Input: dimensioned drawing with shaded views. Units: mm. Origin: part minimum x, y, z. A direction names the side the tool comes from. Round coordinates to 2 decimals unless told otherwise and drop trailing zeros. Loops run counter-clockwise (first coordinate to the right, second up) from the corner with the lowest first, then second, coordinate; pieces in that order, holes last. Notation, with made-up numbers: M 5.5,-29.75 L 54.5,-29.75 A14 ccw 54.5,-14.75 Z; hole C -24,31.5 d3. An arc over 180 degrees is marked long. Use one line per item in the form item = value. Start each with the question number.
Q1. Section query B-B, the plane y = 33. Output: boundary loops of the cut face in (x, z), and give its area (3 significant figures).
Q2. Section query C-C, the plane z = 3.1. Output: boundary loops of the cut face in (x, y), and give its area (3 significant figures).
Q3. First-contact query: P1, Ø3, axis at x = 31.5, z = 2.5, coming from the -Y side; P2, Ø1.5, axis at y = 71.5, z = 3, coming from the -X side; P3, Ø2.5, axis at x = 38, z = 1.5, coming from the -Y side. Flat tips, straight axial feed; report the tip coordinate or a pass-through.
Q4. Ray query, line 1 along Y through (x, z) = (17.5, 3.9); line 2 along Y through (x, z) = (14, 2.7); line 3 along X through (y, z) = (36, 1.95). Return the intervals inside material, ascending.
Q5. Section query D-D, the plane y = 20. Output: boundary loops of the cut face in (x, z).
Q6. Section query A-A, the plane x = 17.5. Output: boundary loops of the cut face in (y, z), and give its area (3 significant figures).
Q7. Access query for the marked faces 1, 2, 3, 4 and 5. Directions: +Z, -Z, +X, -X, +Y, -Y. A direction counts if a zero-diameter tool reaches every point of the face in a straight line with its end or side. Return the directions, or none.
Q8. Mould query, pull axis X, two halves, no side actions, for the marked faces 6, 7 and 8. Classes: pulls with the +X half, pulls with the -X half, needs draft (parallel to the pull), parting line crosses it, or undercut.
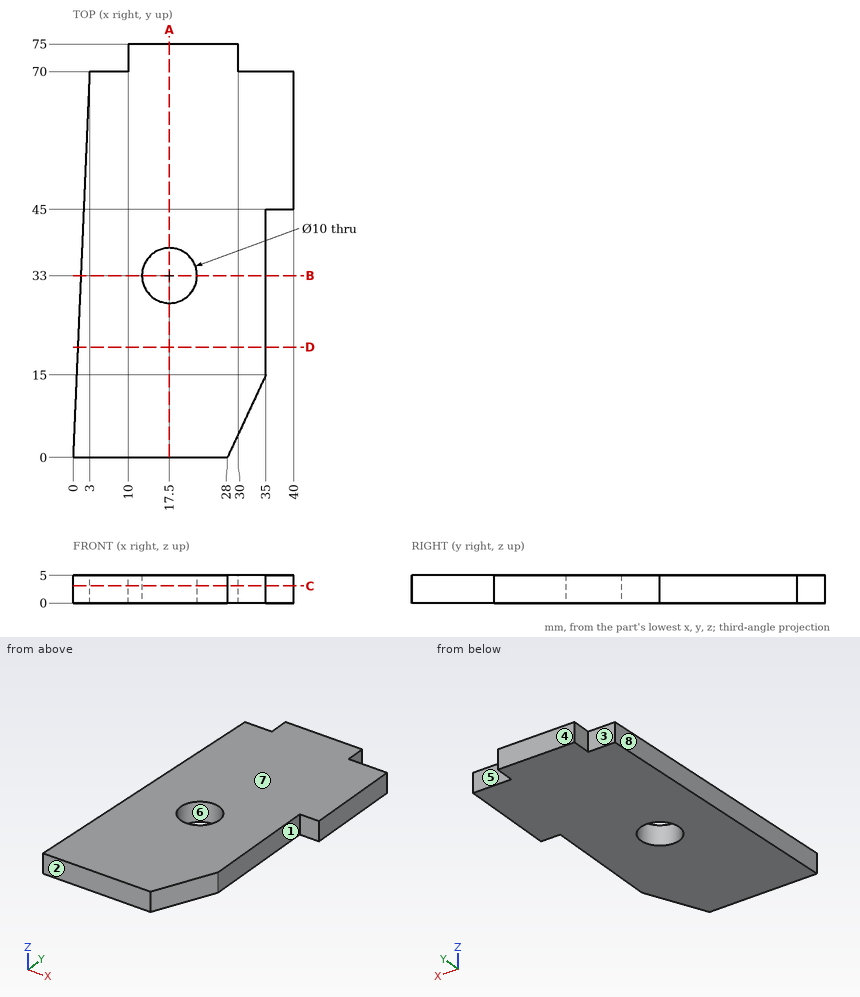
Results found:
q1.outline = M 1.41,0 L 12.5,0 L 12.5,5 L 1.41,5 Z; M 22.5,0 L 35,0 L 35,5 L 22.5,5 Z
q1.area = 118 mm²
q2.outline = M 0,0 L 28,0 L 35,15 L 35,45 L 40,45 L 40,70 L 30,70 L 30,75 L 10,75 L 10,70 L 3,70 Z; hole C 17.5,33 d10
q2.area = 2,440 mm²
q3.P1 = 4.29
q3.P2 = 10
q3.P3 = 45
q4.line_1 = 0 to 28, 38 to 75
q4.line_2 = 0 to 29.43, 36.57 to 75
q4.line_3 = 1.54 to 13.5, 21.5 to 35
q5.outline = M 0.86,0 L 35,0 L 35,5 L 0.86,5 Z
q6.outline = M 0,0 L 28,0 L 28,5 L 0,5 Z; M 38,0 L 75,0 L 75,5 L 38,5 Z
q6.area = 325 mm²
q7.face_1 = +Z, -Z, +X, -Y
q7.face_2 = +Z, -Z, +X, -X, -Y
q7.face_3 = +Z, -Z, -X, +Y
q7.face_4 = +Z, -Z, +X, -X, +Y
q7.face_5 = +Z, -Z, +X, +Y
q8.face_6 = undercut
q8.face_7 = needs draft
q8.face_8 = pulls with the -X half
